Check sheet for the drawn part. Datum: minimum x, y, z corner. Units: mm. A direction names the side the tool comes from. Give positions to 0.01 mm unless a question says otherwise; leave off trailing zeros. Order: outer loops, then holes, each group sorted by start corner. A loop starts at its lowest first (then second) coordinate and runs counter-clockwise, first axis right, second up. Notation, with made-up numbers: (50, 4) - (87, 4) arc R10 cw to (87, 19) - close; hole circle Ø9 at (-19, -27). An arc over 180 degrees is marked (long way). Answer as a JSON object with one key per item and string values. Group by question number.
(1) Section check C-C (x = 5.5). Record the boundary of the cut face in (y, z).
(2) Thickness scan on line 1 (X direction, y = 6, z = 25); line 2 (X direction, y = 15.75, z = 5.5); line 3 (Z direction, x = 4.5, y = 26). Record the ranges inside material, lowest first.
(3) Section check A-A (y = 14). Record the boundary of the cut face in (x, z), then the cut area to 3 significant figures.
(4) Access from +Z, -Z, +X, -X, +Y, -Y to the whole of each face (thin tool, end or side, straight path). Record for the marked faces 4 and 5.
(5) Depth check by flat-ended pin: pin 1 Ø3 at (y, z) = (13, 24.5) entering from +X; pin 2 Ø6.5 at (y, z) = (24, 15.5) entering from +X; pin 3 Ø1.5 at (x, y) = (8, 13) entering from +Z. Enter the tip coordinate at first touch or a pass-through.
(6) Mould release check, pull along Y, two halves, no side actions. Record for the marked faces 1, 2 and 3: +Y half, -Y half, draft (parallel to the pull), parting line (faces both ways), or undercut.
(7) Section check D-D (y = 24). Record the boundary of the cut face in (x, z).
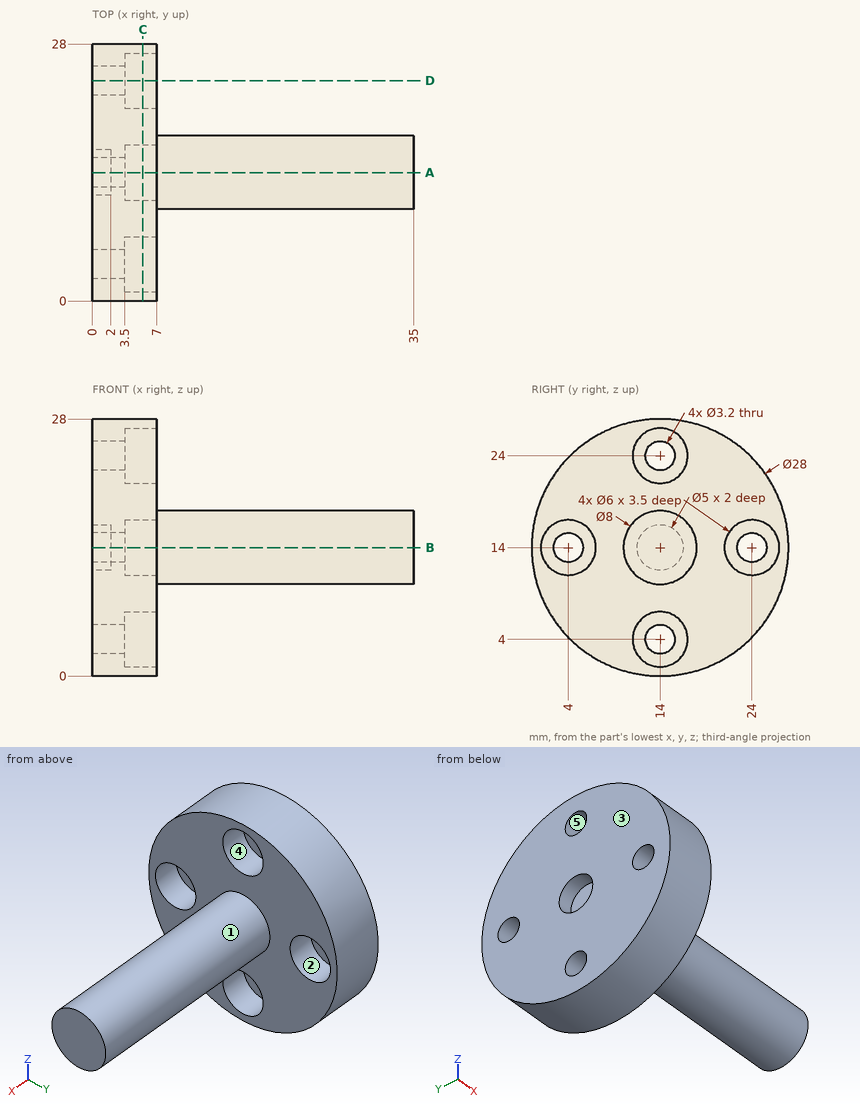
Solutions:
{
 "1": {"outline": "circle Ø28 at (14, 14); hole circle Ø6 at (4, 14); hole circle Ø6 at (14, 4); hole circle Ø6 at (14, 24); hole circle Ø6 at (24, 14)"},
 "2": {"line 1": "x = 0 to 7", "line 2": "x = 0 to 3.5", "line 3": "z = 6.79 to 11.76, 16.24 to 21.21"},
 "3": {"outline": "(0, 0) - (7, 0) - (7, 1) - (3.5, 1) - (3.5, 2.4) - (0, 2.4) - close; (0, 5.6) - (3.5, 5.6) - (3.5, 7) - (7, 7) - (7, 10) - (35, 10) - (35, 18) - (7, 18) - (7, 21) - (3.5, 21) - (3.5, 22.4) - (0, 22.4) - (0, 16.5) - (2, 16.5) - (2, 11.5) - (0, 11.5) - close; (0, 25.6) - (3.5, 25.6) - (3.5, 27) - (7, 27) - (7, 28) - (0, 28) - close", "area": "346 mm2"},
 "4": {"face 4": "+X", "face 5": "+X, -X"},
 "5": {"pin 1": "stops at x = 3.5", "pin 2": "stops at x = 7", "pin 3": "stops at z = 17.99"},
 "6": {"face 1": "parting line", "face 2": "undercut", "face 3": "draft"},
 "7": {"outline": "(0, 4.2) - (7, 4.2) - (7, 11) - (3.5, 11) - (3.5, 12.4) - (0, 12.4) - close; (0, 15.6) - (3.5, 15.6) - (3.5, 17) - (7, 17) - (7, 23.8) - (0, 23.8) - close"}
}
